Answer from the drawing. Dimensions are ordinates in mm from the lowest x, y and z of the part. A direction names the side the tool comes from. Give positions to 0.01 mm unless a question says otherwise; leave off trailing zeros. Loops run counter-clockwise (first coordinate to the right, second up) from the corner with the lowest first, then second, coordinate; pieces in that order, holes last. Notation, with made-up numbers: M -2,47.25 L 15,47.25 A19 ccw 15,63.25 Z; hole C 42,85.5 d6. An arc over 180 degrees is marked long. Return JSON: item names as keys, results as strings. Group by question number.
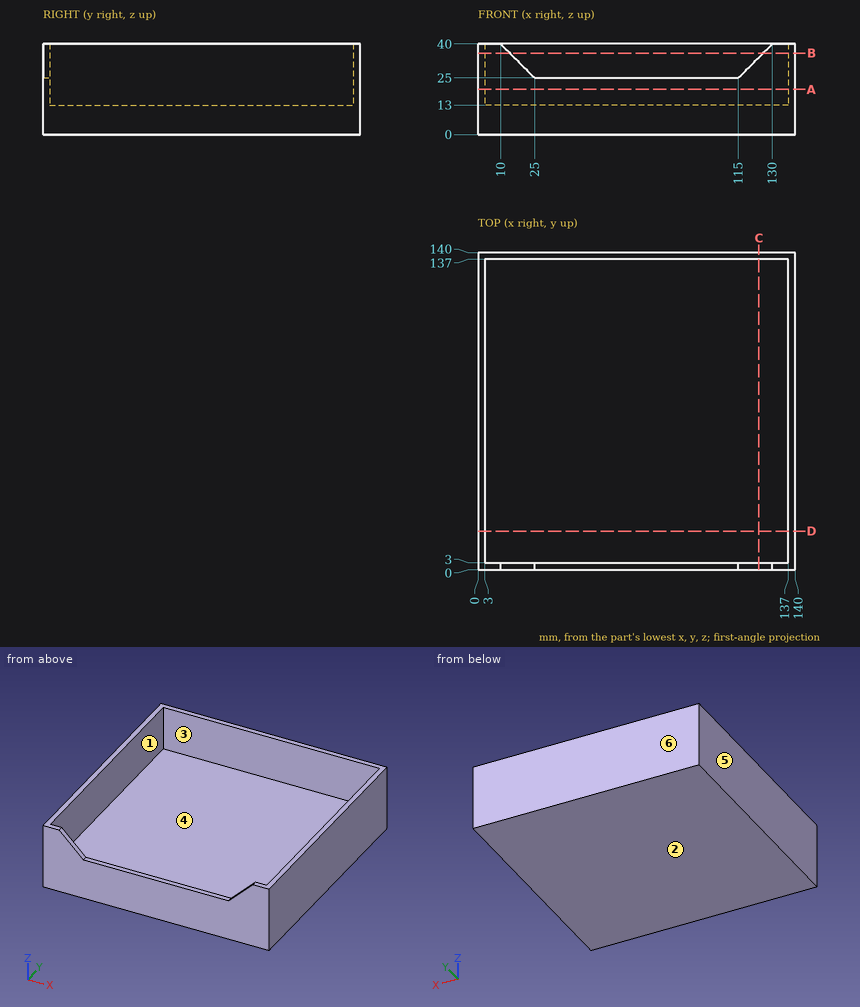
1. Find section B-B (z = 36). Write down the section's boundary in (x, y), and give its area (3 significant figures).
2. Find section D-D (y = 17). Write down the section's boundary in (x, z).
3. For the marked faces 1 and 2, determine the directions among +Z, -Z, +X, -X, +Y, -Y from which every point of the face is accessible in a straight line to the end or side of a thin tool.
4. A flat-ended cylindrical pin translates along its axis: P1, Ø1.5, axis at x = 87, y = 1.5, coming from the +Z side. Find the tip coordinate at first contact, or state that the pin passes through.
5. Straight lines are drawn through the part: line 1 along X through (y, z) = (30.5, 17); line 2 along Z through (x, y) = (123, 99). For each, find the intervals that lie inside material, in ascending order.
6. Find section C-C (x = 124). Write down the section's boundary in (y, z), and give its area (3 significant figures).
7. Find section A-A (z = 20). Write down the section's boundary in (x, y), and give its area (3 significant figures).
8. The mould has two halves that part along X. Classify the marked faces 3, 4, 5 and 6: +X half, -X half, draft (parallel to the pull), parting line (faces both ways), or undercut.
Result:
{
 "1": {"outline": "M 0,0 L 14,0 L 14,3 L 3,3 L 3,137 L 137,137 L 137,3 L 126,3 L 126,0 L 140,0 L 140,140 L 0,140 Z", "area": "1,310 mm2"},
 "2": {"outline": "M 0,0 L 140,0 L 140,40 L 137,40 L 137,13 L 3,13 L 3,40 L 0,40 Z"},
 "3": {"face 1": "+Z", "face 2": "-Z, +X, -X, +Y, -Y"},
 "4": {"P1": "stops at z = 25"},
 "5": {"line 1": "x = 0 to 3, 137 to 140", "line 2": "z = 0 to 13"},
 "6": {"outline": "M 0,0 L 140,0 L 140,40 L 137,40 L 137,13 L 3,13 L 3,34 L 0,34 Z", "area": "1,960 mm2"},
 "7": {"outline": "M 0,0 L 140,0 L 140,140 L 0,140 Z; hole M 3,3 L 137,3 L 137,137 L 3,137 Z", "area": "1,640 mm2"},
 "8": {"face 3": "undercut", "face 4": "undercut", "face 5": "-X half", "face 6": "draft"}
}
